from build123d import *

# Parameters (mm, degrees)
F0_W     = 1.6891
F0_H     = 1.56845
F0_H_2   = 1.6891
F0_W_2   = 1.56845
F1_DEPTH = 15.875
F2_R     = 2.54
F3_DEPTH = 3.96875


with BuildPart() as f1:
    # F0 (on Top) → F1 (new body, symmetric)
    with BuildSketch(Plane.XY):
        with Locations((0, -1.628775)):
            Rectangle(F0_W, F0_H)
        Rectangle(F0_W, F0_H_2)
        with Locations((1.628775, 0)):
            Rectangle(F0_W_2, F0_H_2)
        with Locations((-1.628775, 0)):
            Rectangle(F0_W_2, F0_H_2)
        with Locations((0, 1.628775)):
            Rectangle(F0_W, F0_H)
    extrude(amount=F1_DEPTH, both=True)

    # F2 (on Top) → F3 (join, symmetric)
    with BuildSketch(Plane.XY):
        Circle(F2_R)
    extrude(amount=F3_DEPTH, both=True)


solid = f1.part
The model under review builds one solid part; all positions refer to its coordinate system, in mm. A direction names the side the tool comes from. Give positions to 0.01 mm unless a question says otherwise; leave off trailing zeros. Write each loop counter-clockwise with the first axis right and the second up, starting at its lowest first coordinate (ties: lowest second). Pieces come first, ordered by that corner, then holes.
1. For P1, Ø1.2, axis at x = -1.5, y = 2, coming from the +Z side; P2, Ø0.5, axis at y = -1.5, z = 5, coming from the +X side; P3, Ø1.2, axis at x = 1.5, y = -1.5, coming from the -Z side, all flat-tipped, find the tip position at first contact; note any pin that passes through.
2. Wall thickness on L1, parallel to Z at x = -1.5, y = -1.9; L2, parallel to Y at x = 2.3, z = 6: over which ranges is each line inside the solid? List them lowest first.
3. Add section A-A, the plane z = -9.5. Write out the cut boundary in (x, y), plus the area to 3 significant figures.
4. Tool access review of faces 1 (the flat face through (2, 0.845, 7)), 2 (the flat face through (-1, -1, -3.969)), 3 (the flat face through (-1, -1, 3.969)): name each direction out of +Z, -Z, +X, -X, +Y, -Y from which nothing blocks a thin tool from reaching the whole face with its end or side.
5. Add section B-B, the plane y = 1.4. Write out the cut boundary in (x, z) (3 decimals).
Worked answers:
1. P1: stops at z = 3.97
1. P2: stops at x = 0.84
1. P3: stops at z = -3.97
2. L1: z = -3.97 to 3.97
2. L2: y = -0.84 to 0.84
3. outline: (-2.41, -0.84) - (-0.84, -0.84) - (-0.84, -2.41) - (0.84, -2.41) - (0.84, -0.84) - (2.41, -0.84) - (2.41, 0.84) - (0.84, 0.84) - (0.84, 2.41) - (-0.84, 2.41) - (-0.84, 0.84) - (-2.41, 0.84) - close
3. area: 13.5 mm2
4. face 1: +X, +Y
4. face 2: -Z, -X, -Y
4. face 3: +Z, -X, -Y
5. outline: (-2.119, -3.969) - (-0.845, -3.969) - (-0.845, -15.875) - (0.845, -15.875) - (0.845, -3.969) - (2.119, -3.969) - (2.119, 3.969) - (0.845, 3.969) - (0.845, 15.875) - (-0.845, 15.875) - (-0.845, 3.969) - (-2.119, 3.969) - close
